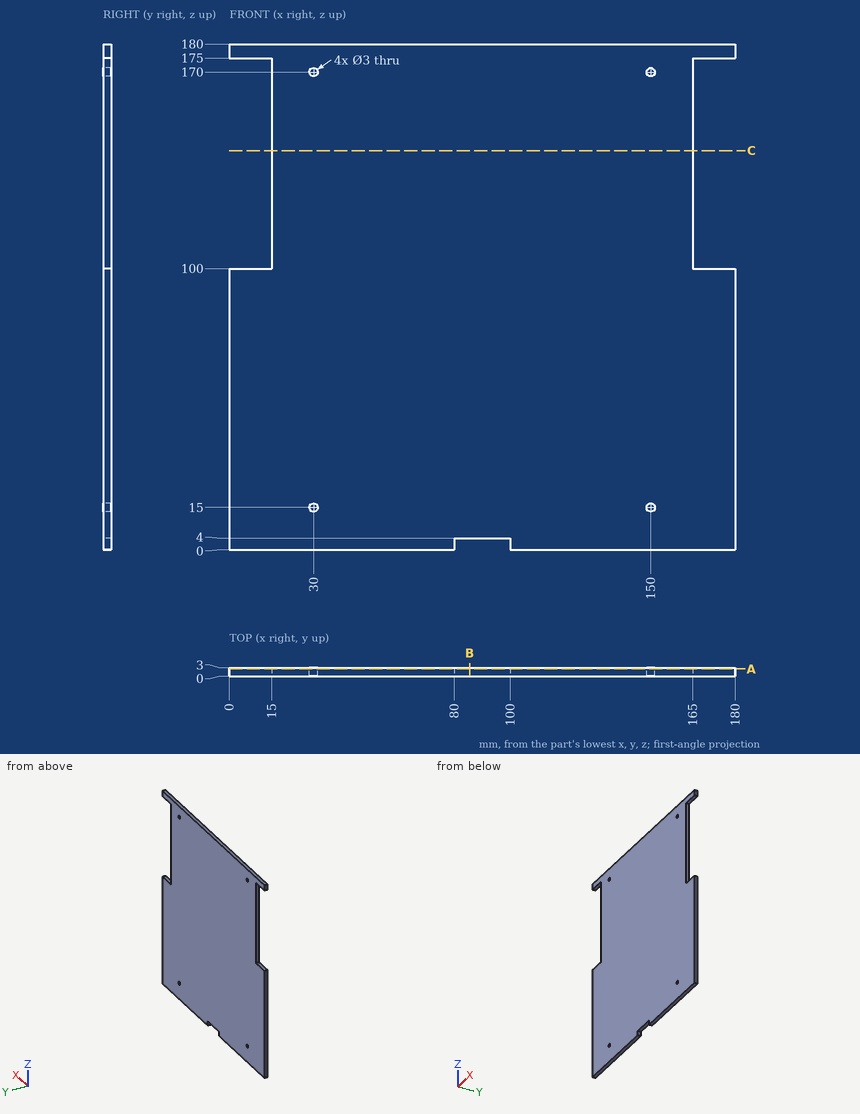
Geometry check sheet. Reference: drawing and pictorial views, mm from the part's lowest x, y, z. Round coordinates to 2 decimals unless told otherwise and drop trailing zeros. Write each loop counter-clockwise with the first axis right and the second up, starting at its lowest first coordinate (ties: lowest second). Pieces come first, ordered by that corner, then holes.
1. Gauge pin test, flat ends, axial feed: P1, Ø0.9, axis at x = 93, y = 2, coming from the -Z side; P2, Ø1.5, axis at y = 2, z = 125, coming from the +X side; P3, Ø12, axis at x = 129, z = 89.5, coming from the -Y side; P4, Ø1.8, axis at x = 30, z = 170, coming from the +Y side. Record the tip position at first contact, or that the pin passes through.
2. Section check B-B on x = 85.5. Enter the section's corners in (y, z), plus the area to 3 significant figures.
3. Section check A-A on y = 2.5. Enter the section's corners in (x, z), plus the area to 3 significant figures.
4. Section check C-C on z = 142. Enter the section's corners in (x, y), plus the area to 3 significant figures.
5. Scan lines: L1, parallel to X at y = 2, z = 15; L2, parallel to Z at x = 150, y = 2.3; L3, parallel to X at y = 1.3, z = 170. Record each from-to range of solid material in increasing order.
Answer:
1. P1: stops at z = 4
1. P2: stops at x = 165
1. P3: stops at y = 0
1. P4: passes through
2. outline: (0, 4) - (3, 4) - (3, 180) - (0, 180) - close
2. area: 528 mm2
3. outline: (0, 0) - (80, 0) - (80, 4) - (100, 4) - (100, 0) - (180, 0) - (180, 100) - (165, 100) - (165, 175) - (180, 175) - (180, 180) - (0, 180) - (0, 175) - (15, 175) - (15, 100) - (0, 100) - close; hole circle Ø3 at (30, 15); hole circle Ø3 at (30, 170); hole circle Ø3 at (150, 15); hole circle Ø3 at (150, 170)
3. area: 30,000 mm2
4. outline: (15, 0) - (165, 0) - (165, 3) - (15, 3) - close
4. area: 450 mm2
5. L1: x = 0 to 28.5, 31.5 to 148.5, 151.5 to 180
5. L2: z = 0 to 13.5, 16.5 to 168.5, 171.5 to 180
5. L3: x = 15 to 28.5, 31.5 to 148.5, 151.5 to 165
